Model file for the job. Use its own axes, mm. A direction names the side the tool comes from. Give positions to 0.01 mm unless a question says otherwise; leave off trailing zeros. Order: outer loops, then holes, each group sorted by start corner. A loop starts at its lowest first (then second) coordinate and runs counter-clockwise, first axis right, second up. Notation, with made-up numbers: (-11.75, 4.5) -> (38.25, 4.5) arc R11 cw to (38.25, 23.5) -> close; hole circle Ø4 at (3.25, 20). An arc over 180 degrees is marked (long way). Use CSV: the item, a comma, the result in double quotes. Start each with the question number.
1. Cut at B-B on x = 0. List the corners of the cut face in (y, z), then the cut area to 3 significant figures.
2. 3-axis set-ups, long thin cutter, end or side, ignore diameter. For faces 4 (the flat face through (-20, 10, 30)), 5 (the flat face through (0, 60, 37.5)), 6 (the flat face through (0, 38, 9)), 7 (the flat face through (-40, 7, 52)), 8 (the flat face through (42, 28, 30)): which of +Z, -Z, +X, -X, +Y, -Y reach the whole face in a straight line?
3. Pull direction X, two halves, no side cores. Call faces 1 (the flat face through (20, 10, 30)), 2 (the flat face through (44, 14, 45)), 3 (the flat face through (-50, 14, 30)): released by +X, released by -X, zero draft, split by the parting line, or undercut.
4. Cut at C-C on y = 26. List the corners of the cut face in (x, z), then the cut area to 3 significant figures.
5. Cut at D-D on x = 24.5. List the corners of the cut face in (y, z).
6. Drop flat-ended pins along their axis: pin 1 (17.5 mm diameter, centred on x = -46, z = 30, fed in from +Y); pin 2 (3 mm diameter, centred on y = 58, z = 44, fed in from -X); pin 3 (2.5 mm diameter, centred on x = -13, z = 57.5, fed in from +Y). Give the stop position or say it passes through.
7. Cut at A-A on z = 30. List the corners of the cut face in (x, y).
8. Wall check: line 1 (Y direction, x = -3.5, z = 29.5); line 2 (X direction, y = 5, z = 55.5); line 3 (Y direction, x = 18, z = 20). Give the ranges that are in metal, low to high. Write a range as from..to.
```python
from build123d import *

# Parameters (mm, degrees)
BOSS_EXTRUDE1_DEPTH      = 60
SKETCH7_W                = 80
SKETCH7_H                = 9
CUT_EXTRUDE4_DEPTH       = 15
SKETCH8_R                = 15
BOSS_EXTRUDE2_DEPTH      = 30
BOSS_EXTRUDE3_DEPTH      = 90
BOSS_EXTRUDE3_DEPTH_BACK = 10
SKETCH10_W               = 30
SKETCH10_H               = 28
SKETCH12_W               = 40
SKETCH12_H               = 20
CUT_EXTRUDE5_DEPTH       = 90
CUT_EXTRUDE6_DEPTH       = 109.282039139
CUT_EXTRUDE6_DEPTH_BACK  = 109.282039139
SKETCH13_W               = 15
SKETCH13_H               = 10


with BuildPart() as part:
    # Sketch1 → Boss-Extrude1 (new body)
    with BuildSketch(Plane.XY):
        Polygon((40, 0), (20, 0), (20, 20), (-20, 20), (-20, 0), (-40, 0), (-40, 15), (-26, 45), (26, 45), (40, 15), align=None)
    extrude(amount=BOSS_EXTRUDE1_DEPTH)

    # Sketch7 → Cut-Extrude4 (cut)
    with BuildSketch(Plane(origin=(0, 45, 0), x_dir=(1, 0, 0), z_dir=(0, 1, 0))):
        with Locations((0, -4.5)):
            Rectangle(SKETCH7_W, SKETCH7_H)
        with Locations((0, -55.5)):
            Rectangle(SKETCH7_W, SKETCH7_H)
    extrude(amount=-CUT_EXTRUDE4_DEPTH, mode=Mode.SUBTRACT)

    # Sketch8 → Boss-Extrude2 (add)
    with BuildSketch(Plane(origin=(0, 45, 0), x_dir=(1, 0, 0), z_dir=(0, 1, 0))):
        with Locations(Location((0, -30, 0), (0, 0, 270))):
            Circle(SKETCH8_R)
    extrude(amount=BOSS_EXTRUDE2_DEPTH)

    # Sketch10 → Boss-Extrude3 (add, two sides: drawn at the far end of the back side and taken through both)
    with BuildSketch(Plane(origin=(-40, 0, 0), x_dir=(0, 0, -1), z_dir=(1, 0, 0)).offset(-BOSS_EXTRUDE3_DEPTH_BACK)):
        with Locations((-30, 14)):
            Rectangle(SKETCH10_W, SKETCH10_H)
    extrude(amount=BOSS_EXTRUDE3_DEPTH + BOSS_EXTRUDE3_DEPTH_BACK)

    # Sketch12 → Cut-Extrude5 (cut)
    with BuildSketch(Plane(origin=(0, 0, 15), x_dir=(-1, 0, 0), z_dir=(0, 0, -1))):
        with Locations((0, 10)):
            Rectangle(SKETCH12_W, SKETCH12_H)
    extrude(amount=-CUT_EXTRUDE5_DEPTH, mode=Mode.SUBTRACT)

    # Sketch13 → Cut-Extrude6 (cut, two sides: drawn at the far end of the back side and taken through both)
    with BuildSketch(Plane(origin=(0, 0, 0), x_dir=(0, 0, -1), z_dir=(1, 0, 0)).offset(-CUT_EXTRUDE6_DEPTH_BACK)):
        with Locations((-30, 60)):
            Rectangle(SKETCH13_W, SKETCH13_H)
    extrude(amount=CUT_EXTRUDE6_DEPTH + CUT_EXTRUDE6_DEPTH_BACK, mode=Mode.SUBTRACT)


solid = part.part
```
Verdict:
1,outline,"(20, 0) -> (30, 0) -> (30, 9) -> (45, 9) -> (45, 15) -> (75, 15) -> (75, 45) -> (45, 45) -> (45, 51) -> (30, 51) -> (30, 60) -> (20, 60) -> close; hole (55, 22.5) -> (65, 22.5) -> (65, 37.5) -> (55, 37.5) -> close"
1,area,"1,980 mm^2"
2,face 4,"+Z, -Z, -Y"
2,face 5,"+X, -X"
2,face 6,"-Z, +X, -X, +Y"
2,face 7,"+Z, -X, +Y, -Y"
2,face 8,"+Z, -Z, +X, +Y"
3,face 1,"undercut"
3,face 2,"zero draft"
3,face 3,"released by -X"
4,outline,"(-50, 15) -> (-34.87, 15) -> (-34.87, 0) -> (34.87, 0) -> (34.87, 15) -> (50, 15) -> (50, 45) -> (34.87, 45) -> (34.87, 60) -> (-34.87, 60) -> (-34.87, 45) -> (-50, 45) -> close"
4,area,"5,090 mm^2"
5,outline,"(0, 0) -> (30, 0) -> (30, 9) -> (45, 9) -> (45, 51) -> (30, 51) -> (30, 60) -> (0, 60) -> close"
6,pin 1,"y = 28"
6,pin 2,"x = -8.29"
6,pin 3,"y = 30"
7,outline,"(-50, 0) -> (-20, 0) -> (-20, 20) -> (20, 20) -> (20, 0) -> (50, 0) -> (50, 28) -> (33.93, 28) -> (26, 45) -> (15, 45) -> (15, 55) -> (-15, 55) -> (-15, 45) -> (-26, 45) -> (-33.93, 28) -> (-50, 28) -> close; (-15, 65) -> (15, 65) -> (15, 75) -> (-15, 75) -> close"
8,line 1,"20..55, 65..75"
8,line 2,"-40..-20, 20..40"
8,line 3,"20..45"
